Geometry check sheet. Reference: the model listing, model coordinates, mm. A direction names the side the tool comes from. Coordinates: 2 decimals unless noted, no trailing zeros. Write each loop counter-clockwise with the first axis right and the second up, starting at its lowest first coordinate (ties: lowest second). Pieces come first, ordered by that corner, then holes. Notation, with made-up numbers: M 77,83 L 127,83 A17 cw 127,113 Z; hole C 10,7.25 d11. An arc over 180 degrees is marked long. Put each result on its own line as item: value. Start each with the question number.
1) Mould release check, pull along Z, two halves, no side actions. Record for faces 3 (the cylindrical face through (-0.69, -3.1, 3.09)), 4 (the cylindrical face through (-1.231, -2.366, 5.977)), 5 (the flat face through (0, 0, 63.5)), 6 (the flat face through (0, 0, 0)): released by +Z, released by -Z, zero draft, split by the parting line, or undercut.
2) Cross-section at A-A on z = 45.5. Record the cut outline in (x, y) (3 decimals), plus the area to 3 significant figures.
3) Gauge pin test, flat end, axial feed: pin 1 (1 mm diameter, centred on x = 2, z = 30, fed in from -Y). Record the tip position at first contact, or that the pin passes through.
4) Scan lines: line 1 along Z through (x, y) = (2, 2.25); line 2 along Z through (x, y) = (-2.75, -0.75); line 3 along Y through (x, z) = (1.75, 28). Record each from-to range of solid material in increasing order.
5) Set-up check for faces 1 (the cylindrical face through (-1.231, -2.366, 38.463)), 2 (the cylindrical face through (-0.69, -3.1, 47.87)): record each of +Z, -Z, +X, -X, +Y, -Y from which the full face is reachable in a straight line by a thin tool's end or side.
from build123d import *

# Parameters (mm, degrees)
SKETCH1_R           = 3.175
BOSS_EXTRUDE1_DEPTH = 63.5
CHAMFER1_SIZE       = 0.635
CUT_EXTRUDE1_START  = 0.7366
SKETCH2_R           = 3.175
SKETCH2_R_2         = 2.667
CUT_EXTRUDE1_DEPTH  = 0.7366
CUT_EXTRUDE3_START  = 0.7366
SKETCH4_R           = 3.175
SKETCH4_R_2         = 2.667
CUT_EXTRUDE3_DEPTH  = 0.7366
SKETCH5_R           = 3.175
SKETCH5_R_2         = 2.667
CUT_EXTRUDE4_DEPTH  = 0.7366


with BuildPart() as part:
    # Sketch1 → Boss-Extrude1 (new body)
    with BuildSketch(Plane.XY):
        Circle(SKETCH1_R)
    extrude(amount=BOSS_EXTRUDE1_DEPTH)

    # Chamfer1
    chamfer1_edges = [part.edges().sort_by_distance(p)[0] for p in [
        (-3.175, 0, 0),
        (-3.175, 0, 63.5),
    ]]
    chamfer(chamfer1_edges, length=CHAMFER1_SIZE)

    # Sketch2 → Cut-Extrude1 (cut)
    with BuildSketch(Plane(origin=(0, 0, 19.05), x_dir=(-1, 0, 0), z_dir=(0, 0, -1)).offset(CUT_EXTRUDE1_START)):
        Circle(SKETCH2_R)
        Circle(SKETCH2_R_2, mode=Mode.SUBTRACT)
    extrude(amount=-CUT_EXTRUDE1_DEPTH, mode=Mode.SUBTRACT)

    # Sketch4 → Cut-Extrude3 (cut)
    with BuildSketch(Plane(origin=(0, 0, 6.35), x_dir=(-1, 0, 0), z_dir=(0, 0, -1)).offset(CUT_EXTRUDE3_START)):
        Circle(SKETCH4_R)
        Circle(SKETCH4_R_2, mode=Mode.SUBTRACT)
    cut_extrude3 = extrude(amount=-CUT_EXTRUDE3_DEPTH, mode=Mode.SUBTRACT)

    # Mirror6: Cut-Extrude3 across plane
    add(cut_extrude3.mirror(Plane(origin=(0, 0, 31.75), x_dir=(1, 0, 0), z_dir=(0, 0, -1))), mode=Mode.SUBTRACT)

    # Sketch5 → Cut-Extrude4 (cut)
    with BuildSketch(Plane(origin=(0, 0, 38.1), x_dir=(-1, 0, 0), z_dir=(0, 0, -1))):
        Circle(SKETCH5_R)
        Circle(SKETCH5_R_2, mode=Mode.SUBTRACT)
    extrude(amount=-CUT_EXTRUDE4_DEPTH, mode=Mode.SUBTRACT)


solid = part.part
Answer key:
1. face 3: zero draft
1. face 4: undercut
1. face 5: released by +Z
1. face 6: released by -Z
2. outline: C 0,0 d6.35
2. area: 31.7 mm²
3. pin 1: stops at y = -2.8
4. line 1: z = 0.47 to 5.61, 6.35 to 18.31, 19.05 to 38.1, 38.84 to 57.15, 57.89 to 63.03
4. line 2: z = 0.31 to 5.61, 6.35 to 18.31, 19.05 to 38.1, 38.84 to 57.15, 57.89 to 63.19
4. line 3: y = -2.65 to 2.65
5. face 1: none
5. face 2: +Z, -Z
